```python
from build123d import *

# Parameters (mm, degrees)
F0_W      = 63.0582608283
F0_H      = 63.4325034916
F1_DEPTH  = 12.7
F2_R      = 5.08
F4_E1_W   = 8.5344002582
F4_E1_H   = 14.732
F5_DEPTH  = 2.032
F4_E2_W   = 8.5344002582
F4_E2_H   = 14.732
F6_DEPTH  = 2.032
F8_D      = 6.7564
F9_W      = 11.2923893612
F9_H      = 4.2961570434
F10_DEPTH = 7.112
F11_R     = 1.4717045876


with BuildPart() as f1:
    # F0 (on Front) → F1 (new body, symmetric)
    with BuildSketch(Plane.XZ):
        with Locations((-4.5010391623, -6.8866405636)):
            Rectangle(F0_W, F0_H)
    extrude(amount=F1_DEPTH, both=True)

    # F2
    f2_edges = [f1.edges().sort_by_distance(p)[0] for p in [
        (27.028091, -12.7, -6.886641),
        (27.028091, 12.7, -6.886641),
        (-36.03017, 12.7, -6.886641),
        (-36.03017, -12.7, -6.886641),
    ]]
    fillet(f2_edges, radius=F2_R)

    # F4_E1 (on explicit) → F5 (join)
    with BuildSketch(Plane(origin=(-16.1959640682, 4.0732366033, 24.8296111822), x_dir=(0, -1, 0), z_dir=(-1, 0, 0))):
        with Locations((4.2672001291, 7.366)):
            Rectangle(F4_E1_W, F4_E1_H)
    extrude(amount=F5_DEPTH)

    # F4_E2 (on explicit) → F6 (join)
    with BuildSketch(Plane(origin=(6.8857083097, 4.0732364287, 24.8296111822), x_dir=(0, -1, 0), z_dir=(-1, 0, 0))):
        with Locations((4.2672001291, 7.366)):
            Rectangle(F4_E2_W, F4_E2_H)
    extrude(amount=-F6_DEPTH)

    # F8 (through all)
    with Locations(Plane.YZ.offset(8.9177083097)):
        with Locations((0, 34.9955298007)):
            Hole(F8_D / 2)

    # F9 (on face) → F10 (cut)
    with BuildSketch(Plane(origin=(0, 0, -38.6028923094), x_dir=(1, 0, 0), z_dir=(0, 0, -1))):
        with Locations((-3.2546349103, 0.5336764734)):
            Rectangle(F9_W, F9_H)
    extrude(amount=-F10_DEPTH, mode=Mode.SUBTRACT)

    # F11
    f11_edges = [f1.edges().sort_by_distance(p)[0] for p in [
        (-8.90083, 1.614402, -35.046892),
    ]]
    fillet(f11_edges, radius=F11_R)


solid = f1.part
```
Input: part model. Units: mm. Frame: model coordinates. A direction names the side the tool comes from. Coordinates: 2 decimals unless noted, no trailing zeros. Loops run counter-clockwise (first coordinate to the right, second up) from the corner with the lowest first, then second, coordinate; pieces in that order, holes last. Notation, with made-up numbers: M -40,-1.75 L -10,-1.75 A29 ccw -10,28.25 Z; hole C 31,-3.75 d3. An arc over 180 degrees is marked long. Use a Markdown table: item, result. Add a question column.
1) Draft query along Z for faces 1 (the cylindrical face through (7.887, 0.44, 38.345)), 2 (the flat face through (-3, -1, -31.491)), 3 (the cylindrical face through (-17.226, 0.44, 38.345)), 4 (the flat face through (-5, -12.7, -6)). Return one class per face: +Z half, -Z half, draft (parallel to the pull), parting line (faces both ways), or undercut.
2) Line query: L1, parallel to Z at x = 7.3, y = 0; L2, parallel to Z at x = -8.5, y = -7.75; L3, parallel to X at y = -11.5, z = -33.5. Output: solid intervals per line, ascending. Write a range as from..to.
3) Pin query (flat end, axial travel): P1, Ø8, axis at y = 8, z = -14, coming from the +X side; P2, Ø11, axis at y = 0, z = 35, coming from the +X side; P3, Ø0.6, axis at x = 7.5, z = 29.5, coming from the -Y side; P4, Ø2, axis at x = -6, y = -0.5, coming from the -Z side. Return the tip coordinate at first contact, or that it passes through.
4) Set-up query: faces 5 (the flat face through (-17, -4.461, 32)), 6 (the flat face through (8, 4.073, 32)), 7 (the flat face through (-8.901, -1, -35)). Return all of +Z, -Z, +X, -X, +Y, -Y with unobstructed straight access to the full face (end or side cutting, diameter ignored); none if empty.
5) Section B-B, the plane x = 10. Return the cut outline in (y, z).
6) Section A-A, the plane y = 6. Return the cut outline in (x, z).
Answer below:
| question | item | result |
|---|---|---|
| 1 | face 1 | undercut |
| 1 | face 2 | -Z half |
| 1 | face 3 | undercut |
| 1 | face 4 | draft |
| 2 | L1 | -38.6..31.62, 38.37..39.56 |
| 2 | L2 | -38.6..24.83 |
| 2 | L3 | -34.23..25.23 |
| 3 | P1 | x = 27.03 |
| 3 | P2 | x = 8.92 |
| 3 | P3 | y = -4.46 |
| 3 | P4 | z = -31.49 |
| 4 | face 5 | +Z, +X, -X, -Y |
| 4 | face 6 | +Z, +X, -X, +Y |
| 4 | face 7 | -Z |
| 5 | outline | M -12.7,-38.6 L 12.7,-38.6 L 12.7,24.83 L -12.7,24.83 Z |
| 6 | outline | M -36.03,-38.6 L 27.03,-38.6 L 27.03,24.83 L -36.03,24.83 Z |
